For this review, take the finished solid that the model builds, in its own axes (mm). A direction names the side the tool comes from. Coordinates: 2 decimals unless noted, no trailing zeros. Write each loop counter-clockwise with the first axis right and the second up, starting at its lowest first coordinate (ties: lowest second). Pieces come first, ordered by that corner, then holes. Notation, with made-up numbers: M 18.25,52 L 31.25,52 A31 ccw 31.25,76 Z; hole C 13.25,44.25 d5. An arc over 180 degrees is marked long. Return JSON: item names as keys, results as strings.
```python
from build123d import *

# Parameters (mm, degrees)
BOX_W             = 45
BOX_H             = 91.6
BOX_DEPTH         = 3.3
CYLINDER_R        = 1.56
CYLINDER_DEPTH    = 3.3
CYLINDER001_R     = 1.56
CYLINDER001_DEPTH = 3.3


with BuildPart() as part:
    # Box → Box (join)
    with BuildSketch(Plane.XY):
        with Locations((22.5, 45.8)):
            Rectangle(BOX_W, BOX_H)
    extrude(amount=BOX_DEPTH)

    # Cylinder → Cylinder (join)
    with BuildSketch(Plane(origin=(3, 0, 1.55), x_dir=(1, 0, 0), z_dir=(0, -1, 0))):
        Circle(CYLINDER_R)
    extrude(amount=CYLINDER_DEPTH)

    # Cylinder001 → Cylinder001 (join)
    with BuildSketch(Plane(origin=(3, 94.7, 1.55), x_dir=(1, 0, 0), z_dir=(0, -1, 0))):
        Circle(CYLINDER001_R)
    extrude(amount=CYLINDER001_DEPTH)


solid = part.part
```
1. We need section B-B (x = 13). State the section outline as (y, z) points.
Checks:
{"outline": "M 0,0 L 91.6,0 L 91.6,3.3 L 0,3.3 Z"}
2. Wall thickness on L1, parallel to Y at x = 16.5, z = 2.35; L2, parallel to Z at x = 21.5, y = 80.5: over which ranges is each line inside the solid? List them lowest first. Write a range as from..to.
Checks:
{"L1": "0..91.6", "L2": "0..3.3"}
3. We need section A-A (z = 1.55). State the section outline as (x, y) points, plus the area to 3 significant figures.
Checks:
{"outline": "M 0,0 L 1.44,0 L 1.44,-3.3 L 4.56,-3.3 L 4.56,0 L 45,0 L 45,91.6 L 4.56,91.6 L 4.56,94.7 L 1.44,94.7 L 1.44,91.6 L 0,91.6 Z", "area": "4,140 mm2"}
4. For faces 1 (the face through (22, 46, 3.3)), 2 (the face through (4.488, -1.627, 2.019)), 3 (the face through (4.488, 93.073, 2.019)), list the 3-axis set-ups (+Z, -Z, +X, -X, +Y, -Y) from which the entire face can be reached by the end or side of a thin tool; tool diameter is ignored.
Checks:
{"face 1": "+Z, +X, -X, +Y, -Y", "face 2": "-Y", "face 3": "+Y"}
5. Clearance check with flat-ended pins moving along their axes: pin 1 Ø1.6 at (x, z) = (24.5, 1) entering from -Y; pin 2 Ø13.5 at (x, y) = (30.5, 50) entering from -Z; pin 3 Ø1 at (x, z) = (32.5, 2) entering from +Y. State where each tip first meets the part, or that it passes through.
Checks:
{"pin 1": "y = 0", "pin 2": "z = 0", "pin 3": "y = 91.6"}
